Check sheet for the modelled part. Datum: model origin and axes. Units: mm. Face numbers are marked on the shaded views. Give positions to 0.01 mm unless a question says otherwise; leave off trailing zeros. Loops run counter-clockwise (first coordinate to the right, second up) from the corner with the lowest first, then second, coordinate; pieces in that order, holes last. Notation, with made-up numbers: (56.25, 58) -> (114.25, 58) arc R15 ccw to (114.25, 76) -> close; hole circle Ø6 at (81, 23). An arc over 180 degrees is marked (long way). Answer as CSV lines item,"result". Start each with the question number.
(1) Section check C-C on z = 205. Enter the section's corners in (x, y), plus the area to 3 significant figures.
(2) Section check B-B on x = 2.5. State how many separate pieces and enclosed holes the cut face has, plus the area to 3 significant figures.
(3) Section check A-A on y = 176.5. Enter the section's corners in (x, z).
(4) Release check for a two-part mould opening along X. For the marked faces 1 and 2 record: pulls with the +X half, pulls with the -X half, needs draft (parallel to the pull), parting line crosses it, or undercut.
(5) Gauge pin test, flat ends, axial feed: pin 1 Ø3 at (x, z) = (4.5, 326) entering from +Y; pin 2 Ø3 at (x, z) = (3.5, 89.5) entering from -Y; pin 3 Ø3 at (x, y) = (3.5, -5.5) entering from +Z; pin 4 Ø12 at (y, z) = (261.5, 286) entering from -X. Record the tip position at first contact, or that the pin passes through.
(6) Material ranges on line 1 (Y direction, x = 6, z = 177); line 2 (Z direction, x = 4.25, y = 260.43); line 3 (Z direction, x = 5.25, y = 188.43), recorded low to high. Write a range as from..to.
from build123d import *

# Parameters (mm, degrees)
SKETCH_R   = 3
SKETCH_W   = 59.8
SKETCH_H   = 10
SKETCH_W_2 = 10
SKETCH_H_2 = 69.8
PAD_DEPTH  = 10


with BuildPart() as part:
    # Sketch → Pad (new body)
    with BuildSketch(Plane.YZ):
        Polygon((0, 0), (0, 30.83), (-10, 30.83), (-10, 80.83), (0, 80.83), (0, 140.1), (-10, 140.1), (-10, 190.1), (0, 190.1), (0, 239.9), (-10, 239.9), (-10, 289.9), (0, 289.9), (0, 345), (400, 345), (400, 289.9), (410, 289.9), (410, 239.9), (400, 239.9), (400, 190.1), (410, 190.1), (410, 140.1), (400, 140.1), (400, 80.83), (410, 80.83), (410, 30.83), (400, 30.83), (400, 0), align=None)
        with Locations((188.43, 6.65)):
            Circle(SKETCH_R, mode=Mode.SUBTRACT)
        with Locations((260.43, 6.65)):
            Circle(SKETCH_R, mode=Mode.SUBTRACT)
        with Locations((260.43, 78.65)):
            Circle(SKETCH_R, mode=Mode.SUBTRACT)
        with Locations((188.43, 78.65)):
            Circle(SKETCH_R, mode=Mode.SUBTRACT)
        with Locations((80.2, 90)):
            Rectangle(SKETCH_W, SKETCH_H, mode=Mode.SUBTRACT)
        with Locations((200, 90)):
            Rectangle(SKETCH_W, SKETCH_H, mode=Mode.SUBTRACT)
        with Locations((319.8, 90)):
            Rectangle(SKETCH_W, SKETCH_H, mode=Mode.SUBTRACT)
        with Locations((165, 282.5)):
            Rectangle(SKETCH_W_2, SKETCH_H_2, mode=Mode.SUBTRACT)
        with Locations((165, 152.5)):
            Rectangle(SKETCH_W_2, SKETCH_H_2, mode=Mode.SUBTRACT)
        with BuildLine():
            ThreePointArc((191.702727, 65.648383), (184.43, 42.65), (191.702727, 19.651617))
            Line((191.702727, 19.651617), (191.702727, 65.648383))
        make_face(mode=Mode.SUBTRACT)
        with BuildLine():
            Line((198.975455, 11.794431), (198.975455, 73.505569))
            ThreePointArc((206.248182, 78.278942), (202.481667, 76.090554), (198.975455, 73.505569))
            Line((206.248182, 7.021058), (206.248182, 78.278942))
            ThreePointArc((198.975455, 11.794431), (202.481667, 9.209446), (206.248182, 7.021058))
        make_face(mode=Mode.SUBTRACT)
        with BuildLine():
            Line((213.520909, 4.166345), (213.520909, 81.133655))
            ThreePointArc((220.793636, 82.484368), (217.125983, 81.977488), (213.520909, 81.133655))
            Line((220.793636, 2.815632), (220.793636, 82.484368))
            ThreePointArc((213.520909, 4.166345), (217.125983, 3.322512), (220.793636, 2.815632))
        make_face(mode=Mode.SUBTRACT)
        with BuildLine():
            Line((228.066364, 2.815632), (228.066364, 82.484368))
            ThreePointArc((235.339091, 81.133655), (231.734017, 81.977488), (228.066364, 82.484368))
            Line((235.339091, 4.166345), (235.339091, 81.133655))
            ThreePointArc((228.066364, 2.815632), (231.734017, 3.322512), (235.339091, 4.166345))
        make_face(mode=Mode.SUBTRACT)
        with BuildLine():
            Line((242.611818, 7.021058), (242.611818, 78.278942))
            ThreePointArc((249.884545, 73.505569), (246.378333, 76.090554), (242.611818, 78.278942))
            Line((249.884545, 73.505569), (249.884545, 11.794431))
            ThreePointArc((242.611818, 7.021058), (246.378333, 9.209446), (249.884545, 11.794431))
        make_face(mode=Mode.SUBTRACT)
        with BuildLine():
            Line((257.157273, 19.651617), (257.157273, 65.648383))
            ThreePointArc((257.157273, 19.651617), (264.43, 42.65), (257.157273, 65.648383))
        make_face(mode=Mode.SUBTRACT)
    extrude(amount=PAD_DEPTH)


solid = part.part
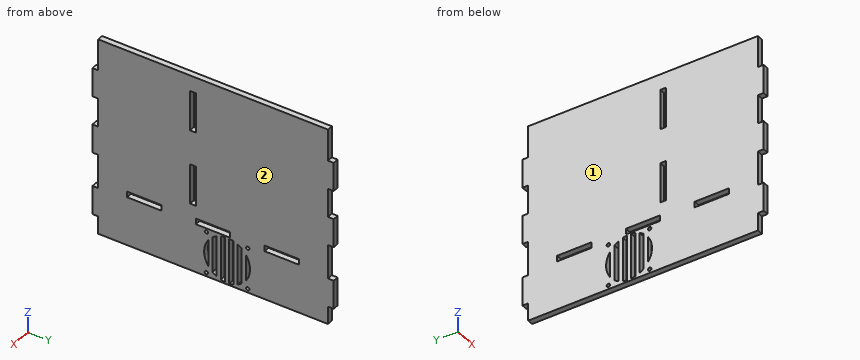
Working result:
1,outline,"(0, 0) -> (10, 0) -> (10, 400) -> (0, 400) -> close"
1,area,"4,000 mm^2"
2,separate pieces,"1"
2,enclosed holes,"15"
2,area,"135,000 mm^2"
3,outline,"(0, 0) -> (10, 0) -> (10, 85) -> (0, 85) -> close; (0, 95) -> (10, 95) -> (10, 345) -> (0, 345) -> close"
4,face 1,"pulls with the -X half"
4,face 2,"pulls with the +X half"
5,pin 1,"stops at y = 400"
5,pin 2,"stops at y = 0"
5,pin 3,"stops at z = 289.9"
5,pin 4,"stops at x = 0"
6,line 1,"y = -10..160, 170..410"
6,line 2,"z = 0..3.65, 9.65..25.21, 60.09..75.65, 81.65..345"
6,line 3,"z = 0..3.65, 9.65..25.21, 60.09..75.65, 81.65..85, 95..345"
